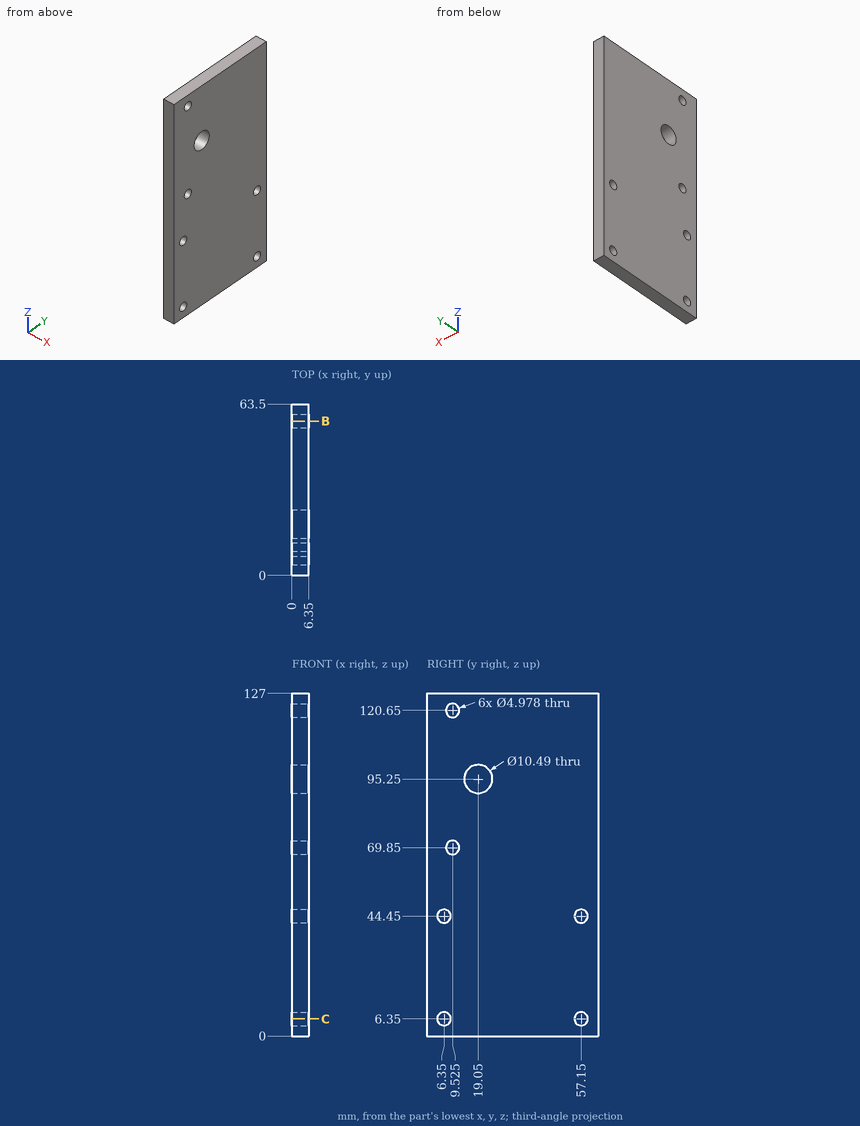
For this review, use the dimensioned drawing (mm, ordinates from the lowest corner) and the shaded views. Coordinates: 2 decimals unless noted, no trailing zeros. Order: outer loops, then holes, each group sorted by start corner. A loop starts at its lowest first (then second) coordinate and runs counter-clockwise, first axis right, second up. Notation, with made-up numbers: (-37, 19.25) - (-30, 19.25) arc R15 cw to (-30, 23.25) - close; hole circle Ø3 at (-37.5, 31.5). An arc over 180 degrees is marked (long way). Answer as a JSON object with one key per item and string values. Group by question number.
1. For probe 1 along Y at (x, z) = (4.75, 6.35); probe 2 along Z at (x, y) = (3.75, 6) (1 decimal); probe 3 along Y at (x, z) = (4.25, 120.65) (1 decimal), list the stretches that pass through material, from the lowest coordinate up.
2. We need section C-C on z = 6.35. State the section outline as (x, y) points, then the cut area to 3 significant figures.
3. We need section B-B on y = 57.15. State the section outline as (x, z) points.
4. Clearance check with a flat-ended pin moving along its axis: P1, Ø4.5, axis at y = 6.35, z = 44.45, coming from the +X side. State where the tip first meets the part, or that it passes through.
Final values:
{
 "1": {"probe 1": "0 to 3.86, 8.84 to 54.66, 59.64 to 63.5", "probe 2": "0 to 3.9, 8.8 to 42, 46.9 to 127", "probe 3": "0 to 7, 12 to 63.5"},
 "2": {"outline": "(0, 0) - (6.35, 0) - (6.35, 3.86) - (0, 3.86) - close; (0, 8.84) - (6.35, 8.84) - (6.35, 54.66) - (0, 54.66) - close; (0, 59.64) - (6.35, 59.64) - (6.35, 63.5) - (0, 63.5) - close", "area": "340 mm²"},
 "3": {"outline": "(0, 0) - (6.35, 0) - (6.35, 3.86) - (0, 3.86) - close; (0, 8.84) - (6.35, 8.84) - (6.35, 41.96) - (0, 41.96) - close; (0, 46.94) - (6.35, 46.94) - (6.35, 127) - (0, 127) - close"},
 "4": {"P1": "through"}
}
